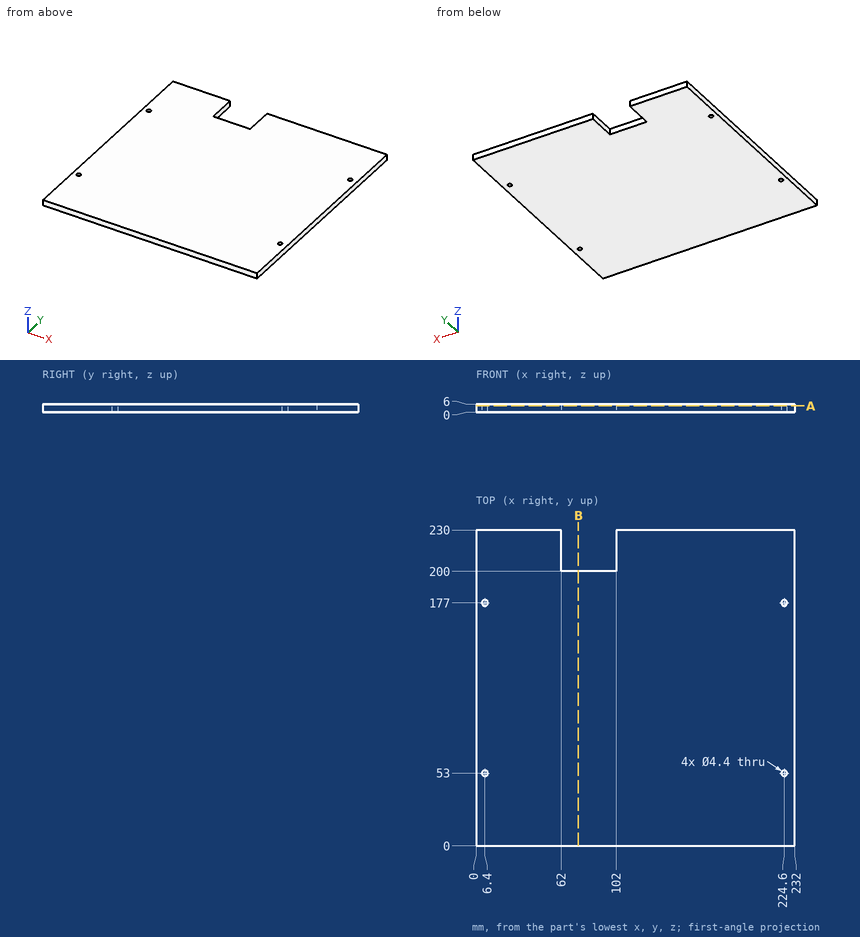
Geometry check sheet. Reference: drawing and pictorial views, mm from the part's lowest x, y, z. Round coordinates to 2 decimals unless told otherwise and drop trailing zeros. Loops run counter-clockwise (first coordinate to the right, second up) from the corner with the lowest first, then second, coordinate; pieces in that order, holes last. Notation, with made-up numbers: (3, 71) - (50, 71) arc R17 cw to (50, 89) - close; hole circle Ø11 at (-17, -1.75). An arc over 180 degrees is marked (long way). Answer as CSV lines item,"result".
(1) Material ranges on line 1 along X through (y, z) = (177, 2.45); line 2 along Y through (x, z) = (6.4, 2.4); line 3 along Y through (x, z) = (97.5, 5.7), recorded low to high.
Output values:
line 1,"x = 0 to 4.2, 8.6 to 222.4, 226.8 to 232"
line 2,"y = 0 to 50.8, 55.2 to 174.8, 179.2 to 230"
line 3,"y = 0 to 200"
(2) Cross-section at B-B, the plane x = 74.5. Enter the section's corners in (y, z).
Output values:
outline,"(0, 0) - (200, 0) - (200, 6) - (0, 6) - close"
(3) Cross-section at A-A, the plane z = 4.55. Enter the section's corners in (x, y), and give its area (3 significant figures).
Output values:
outline,"(0, 0) - (232, 0) - (232, 230) - (102, 230) - (102, 200) - (62, 200) - (62, 230) - (0, 230) - close; hole circle Ø4.4 at (6.4, 53); hole circle Ø4.4 at (6.4, 177); hole circle Ø4.4 at (224.6, 53); hole circle Ø4.4 at (224.6, 177)"
area,"52,100 mm²"
